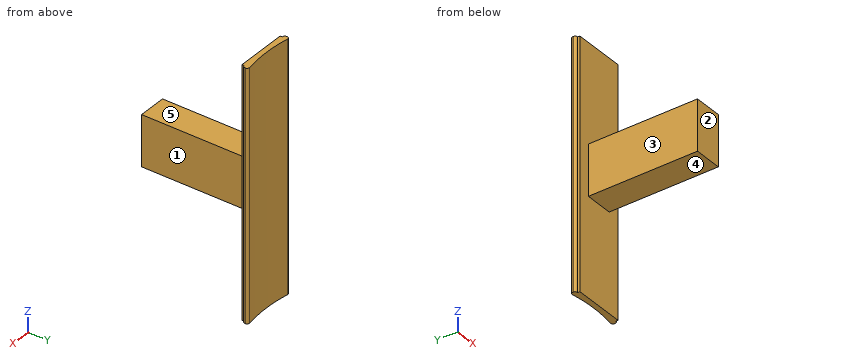
Autodesk Inventor part; units mm, degrees
ref_plane "YZ Plane" through (0, 0, 0) normal (1, 0, 0) x (0, 1, 0)
ref_plane "XZ Plane" through (0, 0, 0) normal (0, 1, 0) x (-1, 0, 0)
ref_plane "XY Plane" through (0, 0, 0) normal (0, 0, 1) x (1, 0, 0)
sketch "Sketch1" plane through (0, 0, 0) normal (0, 0, 1) x (1, 0, 0)
  line L0 (-250, -15) -> (250, -15)
  line L1 (250, -15) -> (250, 35)
  line L2 (-250, 35) -> (-250, -15)
  line L3 (-250, -15) -> (250, 35) construction
  line L4 (250, -15) -> (-250, 35) construction
  arc A0 (-250, 35) -> (250, 35) centre (0, 1314.7822) ccw
  point P0 (0, 10)
  dimension "d6" = 500
  dimension "d7" = 50
extrude "Extrusion1" add sketch "Sketch1" along normal blind 2200
fillet "Fillet1" radius 20 1 edges at (250, 35, 1100)
fillet "Fillet2" radius 20 1 edges at (250, -15, 1100)
fillet "Fillet3" radius 20 2 edges at (-250, 35, 1100) (-250, -15, 1100)
sketch "Sketch2" plane through (230, -15, 0) normal (0, -1, 0) x (1, 0, 0)
  line L0 (0, 2200) -> (0, 0)
  line L1 (-456.5256, 0) -> (-3.4744, 0)
  line L2 (0, 2200) -> (-456.5256, 2200)
  line L3 (-456.5256, 2200) -> (-456.5256, 0)
  line L4 (-456.5256, 0) -> (0, 0)
  line L5 (0, 0) -> (0, 2200)
  line L6 (-103.2628, 1325) -> (-353.2628, 1325)
  line L7 (-353.2628, 1325) -> (-353.2628, 875)
  line L8 (-353.2628, 875) -> (-103.2628, 875)
  line L9 (-103.2628, 875) -> (-103.2628, 1325)
  line L10 (-103.2628, 1325) -> (-353.2628, 875) construction
  line L11 (-353.2628, 1325) -> (-103.2628, 875) construction
  point P0 (-230, 0)
  point P1 (-228.2628, 1100)
  dimension "d15" = 250
  dimension "d16" = 450
extrude "Extrusion2" add sketch "Sketch2" along normal blind 20 contours L0 L4 L1 L3 L2 | L9 L8 L7 L6
sketch "Sketch3" plane through (230, -35, 0) normal (0, -1, 0) x (1, 0, 0)
  point P0 (-230, 0)
sketch "Sketch4" plane through (230, -35, 0) normal (0, -1, 0) x (1, 0, 0)
  line L0 (-105, 1325) -> (-355, 1325)
  line L1 (-355, 1325) -> (-355, 875)
  line L2 (-355, 875) -> (-105, 875)
  line L3 (-105, 875) -> (-105, 1325)
  line L4 (-105, 1325) -> (-355, 875) construction
  line L5 (-355, 1325) -> (-105, 875) construction
  point P0 (-230, 0)
  point P1 (-230, 1100)
  dimension "d17" = 250
  dimension "d18" = 450
extrude "Extrusion3" add sketch "Sketch4" along normal blind 970
properties part number "Patient_table"
Design review of the part built by this model. Coordinates are the model's own, in mm. Face numbers are marked on the shaded views. A direction names the side the tool comes from. Coordinates: 2 decimals unless noted, no trailing zeros. Order: outer loops, then holes, each group sorted by start corner. A loop starts at its lowest first (then second) coordinate and runs counter-clockwise, first axis right, second up. Notation, with made-up numbers: M 8.25,86 L 45.25,86 A17 ccw 45.25,112 Z; hole C -12.5,-12 d9. An arc over 180 degrees is marked long. Answer as a JSON object with one key per item and string values. Group by question number.
1) Add section C-C, the plane y = -112. Write out the cut boundary in (x, z).
2) Tool access review of the marked faces 1, 2, 3, 4 and 5: name each direction out of +Z, -Z, +X, -X, +Y, -Y from which nothing blocks a thin tool from reaching the whole face with its end or side.
3) Add section A-A, the plane x = 0. Write out the cut boundary in (y, z), then the cut area to 3 significant figures.
4) Add section D-D, the plane z = 1848.5. Write out the cut boundary in (x, y).
5) For pin 1 (4 mm diameter, centred on y = -245, z = 1084, fed in from +X); pin 2 (12 mm diameter, centred on x = -44, y = -749.5, fed in from +Z); pin 3 (16 mm diameter, centred on y = -20.5, z = 1171, fed in from +X), all flat-tipped, find the tip position at first contact; note any pin that passes through.
6) Add section B-B, the plane z = 1041.5. Write out the cut boundary in (x, y).
7) Wall thickness on L1, parallel to X at y = -255, z = 1126; L2, parallel to Z at x = -71.5, y = -229; L3, parallel to Y at x = -144, z = 382: over which ranges is each line inside the solid? List them lowest first.
Computed values:
{
 "1": {"outline": "M -125,875 L 125,875 L 125,1325 L -125,1325 Z"},
 "2": {"face 1": "+Z, -Z, +X, -Y", "face 2": "+Z, -Z, +X, -X, -Y", "face 3": "+Z, -Z, -X, -Y", "face 4": "-Z, +X, -X, -Y", "face 5": "+Z, +X, -X, -Y"},
 "3": {"outline": "M -1005,875 L -35,875 L -35,0 L 10.81,0 L 10.81,2200 L -35,2200 L -35,1325 L -1005,1325 Z", "area": "537,000 mm^2"},
 "4": {"outline": "M -250,5 A20 ccw -230,-15 L -226.53,-15 L -226.53,-35 L 230,-35 L 230,-15 A20 ccw 250,5 L 250,10.94 A20 ccw 226.53,30.64 A1303.97 cw -226.53,30.64 A20 ccw -250,10.94 Z"},
 "5": {"pin 1": "stops at x = 125", "pin 2": "stops at z = 1325", "pin 3": "stops at x = 239.68"},
 "6": {"outline": "M -250,5 A20 ccw -230,-15 L -226.53,-15 L -226.53,-35 L -125,-35 L -125,-1005 L 125,-1005 L 125,-35 L 230,-35 L 230,-15 A20 ccw 250,5 L 250,10.94 A20 ccw 226.53,30.64 A1303.97 cw -226.53,30.64 A20 ccw -250,10.94 Z"},
 "7": {"L1": "x = -125 to 125", "L2": "z = 875 to 1325", "L3": "y = -35 to 18.79"}
}
